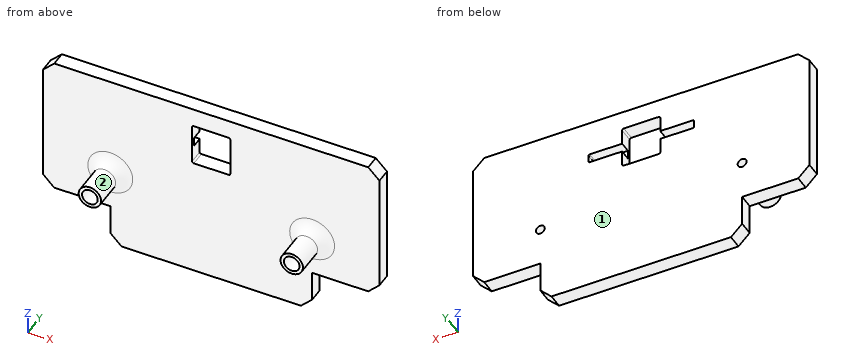
from build123d import *

# Parameters (mm, degrees)
SKETCH1_W           = 150
SKETCH1_H           = 63.315
BOSS_EXTRUDE1_DEPTH = 6.5
SKETCH3_W           = 30
SKETCH3_H           = 6.5
CUT_EXTRUDE1_DEPTH  = 18.75
CHAMFER1_SIZE       = 5
SKETCH5_R           = 5
BOSS_EXTRUDE3_DEPTH = 17.5
FILLET1_R           = 5
SKETCH6_R           = 3.5
CUT_EXTRUDE2_DEPTH  = 17.5
SKETCH7_R           = 3.5
CUT_EXTRUDE3_DEPTH  = 17.5
SKETCH8_R           = 2
CUT_EXTRUDE4_DEPTH  = 6.5
SKETCH11_W          = 150
SKETCH11_H          = 6.5
BOSS_EXTRUDE4_DEPTH = 19
SKETCH12_W          = 17
SKETCH12_H          = 19
CUT_EXTRUDE5_DEPTH  = 19
SKETCH13_W          = 15
SKETCH13_H          = 4
CUT_EXTRUDE6_DEPTH  = 5
FILLET2_R           = 0.5
FILLET3_R           = 0.75
CHAMFER2_SIZE       = 5


with BuildPart() as part:
    # Sketch1 → Boss-Extrude1 (new body)
    with BuildSketch(Plane(origin=(0, 0, 0), x_dir=(1, 0, 0), z_dir=(0, 1, 0))):
        Rectangle(SKETCH1_W, SKETCH1_H)
    extrude(amount=BOSS_EXTRUDE1_DEPTH)

    # Sketch3 → Cut-Extrude1 (cut)
    with BuildSketch(Plane(origin=(0, 0, -31.6575), x_dir=(-1, 0, 0), z_dir=(0, 0, -1))):
        with Locations((-60, 3.25)):
            Rectangle(SKETCH3_W, SKETCH3_H)
        with Locations((60, 3.25)):
            Rectangle(SKETCH3_W, SKETCH3_H)
    extrude(amount=-CUT_EXTRUDE1_DEPTH, mode=Mode.SUBTRACT)

    # Chamfer1
    chamfer1_edges = [part.edges().sort_by_distance(p)[0] for p in [
        (75, 3.25, -12.9075),
        (45, 3.25, -31.6575),
        (-75, 3.25, -12.9075),
        (-45, 3.25, -31.6575),
    ]]
    chamfer(chamfer1_edges, length=CHAMFER1_SIZE)

    # Sketch5 → Boss-Extrude3 (add)
    with BuildSketch(Plane.XZ):
        with Locations(Location((45, 4.4725, 0), (0, 0, 90))):
            Circle(SKETCH5_R)
        with Locations(Location((-45, 4.4725, 0), (0, 0, 90))):
            Circle(SKETCH5_R)
    extrude(amount=BOSS_EXTRUDE3_DEPTH)

    # Fillet1
    fillet1_edges = [part.edges().sort_by_distance(p)[0] for p in [
        (45, 0, -0.5275),
        (-45, 0, -0.5275),
    ]]
    fillet(fillet1_edges, radius=FILLET1_R)

    # Sketch6 → Cut-Extrude2 (cut)
    with BuildSketch(Plane.XZ.offset(17.5)):
        with Locations(Location((45, 4.4725, 0), (0, 0, 270))):
            Circle(SKETCH6_R)
    extrude(amount=-CUT_EXTRUDE2_DEPTH, mode=Mode.SUBTRACT)

    # Sketch7 → Cut-Extrude3 (cut)
    with BuildSketch(Plane.XZ.offset(17.5)):
        with Locations(Location((-45, 4.4725, 0), (0, 0, 270))):
            Circle(SKETCH7_R)
    extrude(amount=-CUT_EXTRUDE3_DEPTH, mode=Mode.SUBTRACT)

    # Sketch8 → Cut-Extrude4 (cut)
    with BuildSketch(Plane.XZ):
        with Locations(Location((45, 4.4725, 0), (0, 0, 270))):
            Circle(SKETCH8_R)
        with Locations(Location((-45, 4.4725, 0), (0, 0, 270))):
            Circle(SKETCH8_R)
    extrude(amount=-CUT_EXTRUDE4_DEPTH, mode=Mode.SUBTRACT)

    # Sketch11 → Boss-Extrude4 (add)
    with BuildSketch(Plane.XY.offset(31.6575)):
        with Locations((0, 3.25)):
            Rectangle(SKETCH11_W, SKETCH11_H)
    extrude(amount=BOSS_EXTRUDE4_DEPTH)

    # Sketch12 → Cut-Extrude5 (cut)
    with BuildSketch(Plane(origin=(0, 6.5, 0), x_dir=(1, 0, 0), z_dir=(0, 1, 0))):
        with Locations((0, -32.6675)):
            Rectangle(SKETCH12_W, SKETCH12_H)
    extrude(amount=-CUT_EXTRUDE5_DEPTH, mode=Mode.SUBTRACT)

    # Sketch13 → Cut-Extrude6 (cut)
    with BuildSketch(Plane(origin=(0, 6.5, 0), x_dir=(1, 0, 0), z_dir=(0, 1, 0))):
        with Locations((-16, -32.6675)):
            Rectangle(SKETCH13_W, SKETCH13_H)
        with Locations((16, -32.6675)):
            Rectangle(SKETCH13_W, SKETCH13_H)
    extrude(amount=-CUT_EXTRUDE6_DEPTH, mode=Mode.SUBTRACT)

    # Fillet2
    fillet2_edges = [part.edges().sort_by_distance(p)[0] for p in [
        (-23.5, 4, 34.6675),
        (-23.5, 4, 30.6675),
        (23.5, 4, 30.6675),
        (23.5, 4, 34.6675),
    ]]
    fillet(fillet2_edges, radius=FILLET2_R)

    # Fillet3
    fillet3_edges = [part.edges().sort_by_distance(p)[0] for p in [
        (8.5, 3.25, 42.1675),
        (-8.5, 3.25, 42.1675),
        (-8.5, 3.25, 23.1675),
        (8.5, 3.25, 23.1675),
    ]]
    fillet(fillet3_edges, radius=FILLET3_R)

    # Chamfer2
    chamfer2_edges = [part.edges().sort_by_distance(p)[0] for p in [
        (-75, 3.25, 50.6575),
        (75, 3.25, 50.6575),
    ]]
    chamfer(chamfer2_edges, length=CHAMFER2_SIZE)


solid = part.part
Could you check a few things on this model? Use its own coordinates, in mm. Face numbers are marked on the shaded views. Coordinates: 2 decimals unless noted, no trailing zeros. Loops run counter-clockwise (first coordinate to the right, second up) from the corner with the lowest first, then second, coordinate; pieces in that order, holes last.
1. Imagine slicing it at C-C (y = 3.5). Give the number of separate pieces and of enclosed holes in the cut face, and give its area (3 significant figures).
2. Imagine slicing it at A-A (y = -16). Please give me the cut outline in (x, z).
3. Imagine slicing it at D-D (x = -29). Please give me the cut outline in (y, z), and give its area (3 significant figures).
4. We'd pull the mould along X, two halves only. Please class the marked faces 1 and 2: released by +X, released by -X, zero draft, split by the parting line, or undercut.
5. I need wall thicknesses on L1, parallel to X at y = 0.25, z = 27.5; L2, parallel to X at y = -0.5, z = 7; L3, parallel to X at y = -5, z = 3. Which ranges of each line are inside material? Lowest first, please.
6. Imagine slicing it at B-B (x = 17). Please give me the cut outline in (y, z), and give its area (3 significant figures).
7. For P1, Ø4.5, axis at x = 45, z = 4.47, coming from the +Y side; P2, Ø3, axis at y = 3, z = -21, coming from the +X side; P3, Ø4.5, axis at x = -45, z = 4.47, coming from the -Y side; P4, Ø3, axis at y = 4.5, z = -21.5, coming from the -X side, each with a flat end and sliding along its axis, tell me the tip position at first contact or that it passes through.
Computed values:
1. separate pieces: 1
1. enclosed holes: 3
1. area: 10,700 mm2
2. outline: circle Ø10 at (-45, 4.47); circle Ø10 at (45, 4.47); hole circle Ø7 at (-45, 4.47); hole circle Ø7 at (45, 4.47)
3. outline: (0, -31.66) - (6.5, -31.66) - (6.5, 50.66) - (0, 50.66) - close
3. area: 535 mm2
4. face 1: zero draft
4. face 2: undercut
5. L1: x = -75 to -8.5, 8.5 to 75
5. L2: x = -52.4 to -47.42, -42.58 to -37.6, 37.6 to 42.58, 47.42 to 52.4
5. L3: x = -49.78 to -48.18, -41.82 to -40.22, 40.22 to 41.82, 48.18 to 49.78
6. outline: (0, -31.66) - (6.5, -31.66) - (6.5, 30.67) - (1.5, 30.67) - (1.5, 34.67) - (6.5, 34.67) - (6.5, 50.66) - (0, 50.66) - close
6. area: 515 mm2
7. P1: stops at y = 6.5
7. P2: stops at x = 45
7. P3: stops at y = 0
7. P4: stops at x = -45
